For this review, take the finished solid that the model builds, in its own axes (mm). Face numbers are marked on the shaded views. Round coordinates to 2 decimals unless told otherwise and drop trailing zeros. Write each loop counter-clockwise with the first axis right and the second up, starting at its lowest first coordinate (ties: lowest second). Pieces come first, ordered by that corner, then holes. Notation, with made-up numbers: M 7.5,11 L 49.5,11 A31 ccw 49.5,45 Z; hole C 81.25,62 d2. An arc over 180 degrees is marked long. Write each question's results on one line, items separated by ' | '. Start each with the question number.
```python
from build123d import *

# Parameters (mm, degrees)
SKETCH_5_W      = 2.8
SKETCH_5_H      = 8
EXTRUDE_1_DEPTH = 2


with BuildPart() as part:
    # 草图4 → 旋转1 (revolve)
    with BuildSketch(Plane(origin=(0, 0, 0), x_dir=(1, 0, 0), z_dir=(0, 1, 0))):
        with BuildLine():
            Line((0, -3.8), (0, 0))
            Line((0, 0), (-1.4, 0))
            Line((-1.4, 0), (-1.4, -4.625403331))
            ThreePointArc((-1.4, -4.625403331), (-0.812602403, -4.021712173), (0, -3.8))
        make_face()
        with BuildLine():
            Line((-1.4, -6.174596669), (-1.4, -4.625403331))
            ThreePointArc((-1.4, -4.625403331), (-1.6, -5.4), (-1.4, -6.174596669))
        make_face()
        with BuildLine():
            Line((0, -7), (0, -3.8))
            ThreePointArc((0, -3.8), (-0.812602403, -4.021712173), (-1.4, -4.625403331))
            Line((-1.4, -4.625403331), (-1.4, -6.174596669))
            ThreePointArc((-1.4, -6.174596669), (-0.812602403, -6.778287827), (0, -7))
        make_face()
    revolve(axis=Axis((0, 0, -1.647649903), (0, 0, 1)))

    # 草图5 → 凸台-拉伸1 (add)
    with BuildSketch(Plane(origin=(0, 0, 0), x_dir=(-1, 0, 0), z_dir=(0, 0, -1))):
        with Locations((0, 4)):
            Rectangle(SKETCH_5_W, SKETCH_5_H)
    extrude(amount=-EXTRUDE_1_DEPTH)

    # 镜向1: part across plane


with BuildPart() as part_1:
    add(part.part)
    add(part.part.mirror(Plane(origin=(1.4, 8, 2), x_dir=(0, 0, 1), z_dir=(0, 1, 0))))


solid = part_1.part
```
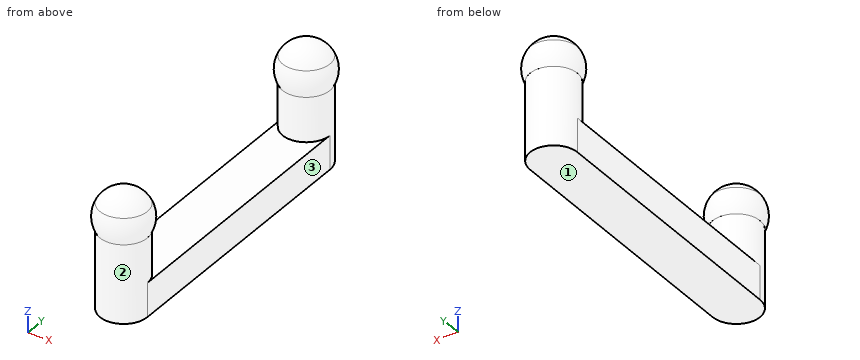
Item 1: We need section A-A on x = 0. State the section outline as (y, z) points.
Item 2: We need section B-B on z = 5.5. State the section outline as (x, y) points, then the cut area to 3 significant figures.
Item 3: Insertion check: P1, Ø1.5, axis at x = 1, y = 9, coming from the +Z side; P2, Ø1.6, axis at y = 10, z = 1, coming from the -X side; P3, Ø0.6, axis at y = 8, z = 0.5, coming from the +X side. Each pin has a flat end and moves straight along its axis. Give the tip position at first contact, or say it passes through.
Item 4: For probe 1 along Z at (x, y) = (-0.65, 11); probe 2 along X at (y, z) = (0.5, 1.5); probe 3 along Y at (x, z) = (1.2, 2.25), list the stretches that pass through material, from the lowest coordinate up.
Item 5: Mouldability with a two-part tool opening along Z and no side actions: class the marked faces 1, 2 and 3 as pulls with the +Z half, pulls with the -Z half, needs draft (parallel to the pull), parting line crosses it, or undercut.
Item 6: We need section D-D on z = 1.5. State the section outline as (x, y) points.
Item 7: We need section C-C on y = 13.75. State the section outline as (x, z) points, then the cut area to 3 significant figures.
Numbers:
1) outline: M -1.4,0 L 17.4,0 L 17.4,4.63 A1.6 ccw long 14.6,4.63 L 14.6,2 L 1.4,2 L 1.4,4.63 A1.6 ccw long -1.4,4.63 Z
2) outline: C 0,0 d3.19; C 0,16 d3.19 | area: 16.0 mm^2
3) P1: stops at z = 2 | P2: stops at x = -1.4 | P3: stops at x = 1.4
4) probe 1: z = 0 to 2 | probe 2: x = -1.4 to 1.4 | probe 3: y = -0.72 to 0.72, 15.28 to 16.72
5) face 1: pulls with the -Z half | face 2: undercut | face 3: needs draft
6) outline: M -1.4,0 A1.4 ccw 1.4,0 L 1.4,16 A1.4 ccw -1.4,16 Z
7) outline: M -1.4,0 L 1.4,0 L 1.4,2 L -1.4,2 Z | area: 5.60 mm^2
